The listing builds one solid part. Answer for the finished solid, in the listing's coordinates (mm). A direction names the side the tool comes from. Coordinates: 2 decimals unless noted, no trailing zeros. Order: outer loops, then holes, each group sorted by start corner. A loop starts at its lowest first (then second) coordinate and runs counter-clockwise, first axis right, second up. Notation, with made-up numbers: (-9, -22) - (25, -22) arc R28 cw to (25, 7) - close; hole circle Ø8 at (6.25, -37). An arc over 180 degrees is marked (long way). Use one line per item in the form item = value. Start each with the question number.
Item 1: Each of these flat-tipped pins is pushed along its axis until it touches: pin 1 Ø3.5 at (x, z) = (25.5, 2.5) entering from +Y; pin 2 Ø1.2 at (x, z) = (15.5, 0.5) entering from -Y. Where does it stop, or does it pass through?
Item 2: The mould has two halves that part along Z. Classify faces 4 (the flat face through (15, 2, 2)), 5 (the flat face through (-31.5, 5, 0)), 6 (the flat face through (0, 5, 6.5)): released by +Z, released by -Z, zero draft, split by the parting line, or undercut.
Item 3: Section C-C, the plane y = 2 is taken. Write down the section's boundary in (x, z), and give its area (3 significant figures).
Item 4: Section B-B, the plane y = 8.5 is taken. Write down the section's boundary in (x, z).
Item 5: Section A-A, the plane x = 0 is taken. Write down the section's boundary in (y, z).
Item 6: A tool of negligible diameter and unlimited length cuts with its end or side. For faces 1 (the cylindrical face through (-2.44, 5.07, -0.54)), 2 (the cylindrical face through (12.5, 2.5, 0)), 3 (the flat face through (-29, 3.2, 0)), from which of +Z, -Z, +X, -X, +Y, -Y can it reach the whole face along a straight path? Write none if from no direction.
Item 7: Consider line 1 along X through (y, z) = (2.2, 0); line 2 along X through (y, z) = (8.5, 4.75); line 3 along X through (y, z) = (8, 0). Determine where each line is inside the solid, lowest interval first. Write a range as [from, to].
Item 8: Section D-D, the plane z = 4 is taken. Write down the section's boundary in (x, y).
from build123d import *

# Parameters (mm, degrees)
SKETCH_1_W                = 63
SKETCH_1_H                = 13
EXTRUDE_1_DEPTH           = 10
HOLE_WIZARD_1_D           = 6.6
HOLE_WIZARD_1_CBORE_D     = 11
HOLE_WIZARD_1_CBORE_DEPTH = 6.8
MM_1_D                    = 4
MM_1_DEPTH                = 5
MM_1_TIP                  = 1.201721238
CUT_EXTRUDE_1_DEPTH       = 5
HOLE_WIZARD_M6_1_D        = 5


with BuildPart() as part:
    # 草图1 → 凸台-拉伸1 (new body)
    with BuildSketch(Plane(origin=(0, 0, 0), x_dir=(1, 0, 0), z_dir=(0, 1, 0))):
        Rectangle(SKETCH_1_W, SKETCH_1_H)
    extrude(amount=EXTRUDE_1_DEPTH)

    # 打孔尺寸(%根据)内六角圆柱头螺钉的类型1 (through all)
    with Locations(Plane(origin=(-25, 10, 0), x_dir=(0, 0, 1), z_dir=(0, 1, 0))):
        with Locations((0, 0), (0, 50)):
            CounterBoreHole(HOLE_WIZARD_1_D / 2, HOLE_WIZARD_1_CBORE_D / 2, HOLE_WIZARD_1_CBORE_DEPTH)

    # 大小mm 暗销孔1
    with Locations(Plane(origin=(-15, 0, 0), x_dir=(0, 0, -1), z_dir=(0, -1, 0))):
        with Locations((0, 0)):
            Hole(MM_1_D / 2, depth=MM_1_DEPTH)
            with Locations((0, 0, -(MM_1_DEPTH + MM_1_TIP / 2))):  # 118° drill point
                Cone(0, MM_1_D / 2, MM_1_TIP, mode=Mode.SUBTRACT)

    # 草图6 → 切除-拉伸1 (cut)
    with BuildSketch(Plane.XZ):
        with BuildLine():
            Line((14.5, 2), (15.5, 2))
            ThreePointArc((15.5, 2), (17.5, 0), (15.5, -2))
            Line((15.5, -2), (14.5, -2))
            ThreePointArc((14.5, -2), (12.5, 0), (14.5, 2))
        make_face()
    extrude(amount=-CUT_EXTRUDE_1_DEPTH, mode=Mode.SUBTRACT)

    # M6 螺纹孔1 (through all)
    with Locations(Plane(origin=(0, 0, 0), x_dir=(0, 0, -1), z_dir=(0, -1, 0))):
        with Locations((0, 0)):
            Hole(HOLE_WIZARD_M6_1_D / 2)


solid = part.part
Response:
q1.pin_1 = 3.2
q1.pin_2 = 5
q2.face_4 = undercut
q2.face_5 = zero draft
q2.face_6 = released by +Z
q3.outline = (-31.5, -6.5) - (31.5, -6.5) - (31.5, 6.5) - (-31.5, 6.5) - close; hole circle Ø6.6 at (-25, 0); hole circle Ø4 at (-15, 0); hole circle Ø5 at (0, 0); hole (14.5, -2) - (15.5, -2) arc R2 ccw to (15.5, 2) - (14.5, 2) arc R2 ccw to start; hole circle Ø6.6 at (25, 0)
q3.area = 702 mm2
q4.outline = (-31.5, -6.5) - (31.5, -6.5) - (31.5, 6.5) - (-31.5, 6.5) - close; hole circle Ø11 at (-25, 0); hole circle Ø5 at (0, 0); hole circle Ø11 at (25, 0)
q5.outline = (0, -6.5) - (10, -6.5) - (10, -2.5) - (0, -2.5) - close; (0, 2.5) - (10, 2.5) - (10, 6.5) - (0, 6.5) - close
q6.face_1 = +Y, -Y
q6.face_2 = -Y
q6.face_3 = +Y
q7.line_1 = [-31.5, -28.3], [-21.7, -17], [-13, -2.5], [2.5, 12.5], [17.5, 21.7], [28.3, 31.5]
q7.line_2 = [-31.5, -27.77], [-22.23, 22.23], [27.77, 31.5]
q7.line_3 = [-31.5, -30.5], [-19.5, -2.5], [2.5, 19.5], [30.5, 31.5]
q8.outline = (-31.5, 0) - (31.5, 0) - (31.5, 10) - (28.77, 10) - (28.77, 3.2) - (21.23, 3.2) - (21.23, 10) - (-21.23, 10) - (-21.23, 3.2) - (-28.77, 3.2) - (-28.77, 10) - (-31.5, 10) - close
